from build123d import *

# Parameters (mm, degrees)
SKETCH1_R           = 35
SKETCH1_R_2         = 25
SKETCH1_R_3         = 1.5
BOSS_EXTRUDE1_DEPTH = 1
FILLET1_R           = 4


with BuildPart() as part:
    # Sketch1 → Boss-Extrude1 (new body)
    # profile 1 of 4: a face of its own
    with BuildSketch(Plane(origin=(0, 0, 0), x_dir=(1, 0, 0), z_dir=(0, 1, 0))):
        Circle(SKETCH1_R)
        with Locations(Location((0, 0, 0), (0, 0, 270))):
            Circle(SKETCH1_R_2, mode=Mode.SUBTRACT)
    # profile 2 of 4: a face of its own
    with BuildSketch(Plane(origin=(0, 0, 0), x_dir=(1, 0, 0), z_dir=(0, 1, 0))):
        with BuildLine():
            ThreePointArc((-20.849440266, 28.11228985), (-17.5, 30.310889132), (-13.921237036, 32.11228985))
            Line((-13.921237036, 32.11228985), (-19.035586192, 40.970602437))
            Line((-19.035586192, 40.970602437), (-19.035898385, 40.97114317))
            ThreePointArc((-19.035898385, 40.97114317), (-24.5, 42.435244785), (-25.964101615, 36.97114317))
            Line((-25.964101615, 36.97114317), (-20.849440266, 28.11228985))
        make_face()
        with Locations(Location((-22.5, 38.97114317, 0), (0, 0, 270))):
            Circle(SKETCH1_R_3, mode=Mode.SUBTRACT)
    # profile 3 of 4: a face of its own
    with BuildSketch(Plane(origin=(0, 0, 0), x_dir=(1, 0, 0), z_dir=(0, 1, 0))):
        with BuildLine():
            Line((-19.035898385, -40.97114317), (-13.921237036, -32.11228985))
            ThreePointArc((-13.921237036, -32.11228985), (-17.5, -30.310889132), (-20.849440266, -28.11228985))
            Line((-20.849440266, -28.11228985), (-25.963789422, -36.970602437))
            Line((-25.963789422, -36.970602437), (-25.964101615, -36.97114317))
            ThreePointArc((-25.964101615, -36.97114317), (-24.5, -42.435244785), (-19.035898385, -40.97114317))
        make_face()
        with Locations(Location((-22.5, -38.97114317, 0), (0, 0, 270))):
            Circle(SKETCH1_R_3, mode=Mode.SUBTRACT)
    # profile 4 of 4: a face of its own
    with BuildSketch(Plane(origin=(0, 0, 0), x_dir=(1, 0, 0), z_dir=(0, 1, 0))):
        with BuildLine():
            ThreePointArc((45, -4), (49, 0), (45, 4))
            Line((45, 4), (34.770677301, 4))
            ThreePointArc((34.770677301, 4), (34.942622294, 2.00328411), (35, 0))
            ThreePointArc((35, 0), (34.942622294, -2.00328411), (34.770677301, -4))
            Line((34.770677301, -4), (44.999375615, -4))
            Line((44.999375615, -4), (45, -4))
        make_face()
        with Locations(Location((45, 0, 0), (0, 0, 270))):
            Circle(SKETCH1_R_3, mode=Mode.SUBTRACT)
    extrude(amount=BOSS_EXTRUDE1_DEPTH)

    # Fillet1
    fillet1_edges = [part.edges().sort_by_distance(p)[0] for p in [
        (-13.921237036, 0.5, 32.11228985),
        (-20.849440266, 0.5, 28.11228985),
        (-20.849440266, 0.5, -28.11228985),
        (-13.921237036, 0.5, -32.11228985),
        (34.770677301, 0.5, -4),
        (34.770677301, 0.5, 4),
    ]]
    fillet(fillet1_edges, radius=FILLET1_R)


solid = part.part
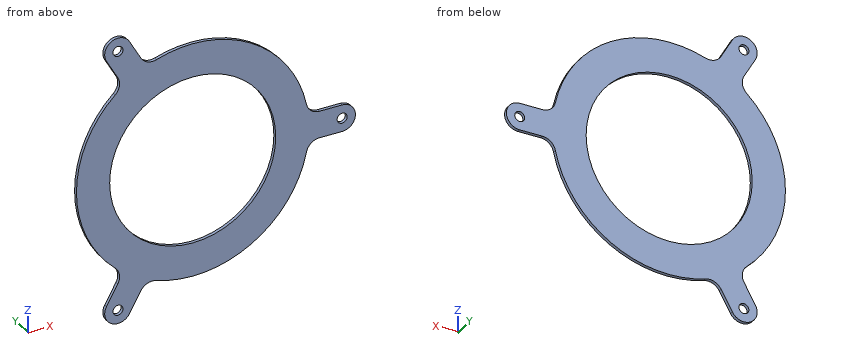
Part model, mm, in its own coordinate system. Give positions to 0.01 mm unless a question says otherwise; leave off trailing zeros. Order: outer loops, then holes, each group sorted by start corner. A loop starts at its lowest first (then second) coordinate and runs counter-clockwise, first axis right, second up. Notation, with made-up numbers: (53.5, -2) - (112.5, -2) arc R15 cw to (112.5, 17) - close; hole circle Ø4 at (63.25, 69.5). An arc over 180 degrees is marked (long way). Use a Markdown table: item, result.
1) Probe L1, parallel to X at y = 0.5, z = 0; L2, parallel to X at y = 0.4, z = 39.5; L3, parallel to X at y = 0.95, z = -22. List the from-to ranges inside material, lowest first. Write a range as from..to.
Checked values:
| item | result |
|---|---|
| L1 | -35..-25, 25..43.5, 46.5..49 |
| L2 | -26.46..-23.9, -21.1..-18.19 |
| L3 | -27.22..-11.87, 11.87..27.22 |
2) Saw through at A-A on z = 0. List the corners of the cut face in (x, y).
Checked values:
| item | result |
|---|---|
| outline | (-35, 0) - (-25, 0) - (-25, 1) - (-35, 1) - close; (25, 0) - (43.5, 0) - (43.5, 1) - (25, 1) - close; (46.5, 0) - (49, 0) - (49, 1) - (46.5, 1) - close |
3) Saw through at D-D on z = -20. List the corners of the cut face in (x, y), plus the area to 3 significant figures.
Checked values:
| item | result |
|---|---|
| outline | (-28.72, 0) - (-15, 0) - (-15, 1) - (-28.72, 1) - close; (15, 0) - (28.72, 0) - (28.72, 1) - (15, 1) - close |
| area | 27.4 mm² |
4) Saw through at B-B on x = -4.5. List the corners of the cut face in (y, z).
Checked values:
| item | result |
|---|---|
| outline | (0, -34.71) - (1, -34.71) - (1, -24.59) - (0, -24.59) - close; (0, 24.59) - (1, 24.59) - (1, 34.71) - (0, 34.71) - close |
5) Saw through at C-C on y = 0.4. Count the separate pieces of the cut face and the enclosed holes in it, plus the area to 3 significant figures.
Checked values:
| item | result |
|---|---|
| separate pieces | 1 |
| enclosed holes | 4 |
| area | 2,190 mm² |
